Work out the finished part from the listing and answer in its coordinate system (mm). A direction names the side the tool comes from. Coordinates: 2 decimals unless noted, no trailing zeros. Order: outer loops, then holes, each group sorted by start corner. A loop starts at its lowest first (then second) coordinate and runs counter-clockwise, first axis right, second up.
1. The part is cut by section A-A, the plane y = -2.15. Give the vertices of the cut face in (x, z) (3 decimals).
2. The part is cut by section C-C, the plane y = -1.15. Give the vertices of the cut face in (x, z) (3 decimals).
3. Flat-ended cylindrical pins translate along their axes: pin 1 Ø2.5 at (x, z) = (-6, -1.5) entering from -Y; pin 2 Ø4 at (x, z) = (-3.5, 2) entering from +Y; pin 3 Ø1.6 at (x, y) = (-4.5, -1) entering from -Z. Find the tip coordinate at first contact, or state that the pin passes through.
4. The part is cut by section D-D, the plane x = -4.5. Give the vertices of the cut face in (y, z).
5. The part is cut by section B-B, the plane z = 1.25. Give the vertices of the cut face in (x, y).
6. A tool of negligible diameter and unlimited length cuts with its end or side. For faces 1 (the flat face through (-9, -1, -0.51)), 2 (the flat face through (-5.915, -1, -4)), 3 (the flat face through (-5.915, -1, 2)), from which of +Z, -Z, +X, -X, +Y, -Y can it reach the whole face along a straight path? Write none if from no direction.
7. Find the intervals of material crossed by probe 1 along Y at (x, z) = (-9.5, -2.25); probe 2 along X at (y, z) = (-1.45, -0.75); probe 3 along X at (y, z) = (-2.7, 0), in increasing order.
```python
from build123d import *

# Parameters (mm, degrees)
F1_DEPTH = 3
F0_W     = 0.8
F0_H     = 0.8
F2_DEPTH = 0.5
F3_DEPTH = 2


with BuildPart() as f1:
    # F0 (on Front) → F1 (new body)
    with BuildSketch(Plane.XZ):
        with BuildLine():
            Line((-6.7150478527, -4.8896004256), (-6.7150478527, -3.377443213))
            ThreePointArc((-6.7150478527, -3.377443213), (-8.0828148057, -2.6774176301), (-8.7828403885, -1.3096506771))
            Line((-8.7828403885, -1.3096506771), (-10.2949976011, -1.3096506771))
            ThreePointArc((-10.2949976011, -1.3096506771), (-9.1434749774, -3.7380778019), (-6.7150478527, -4.8896004256))
        make_face()
        with BuildLine():
            Line((-5.9150478527, -4.8896004256), (-5.9150478527, -3.377443213))
            ThreePointArc((-5.9150478527, -3.377443213), (-6.3150478527, -3.4096506771), (-6.7150478527, -3.377443213))
            Line((-6.7150478527, -3.377443213), (-6.7150478527, -4.8896004256))
            Line((-6.7150478527, -4.8896004256), (-5.9150478527, -4.8896004256))
        make_face()
        with BuildLine():
            Line((-2.3350981043, -1.3096506771), (-3.8472553168, -1.3096506771))
            ThreePointArc((-3.8472553168, -1.3096506771), (-4.5472808997, -2.6774176301), (-5.9150478527, -3.377443213))
            Line((-5.9150478527, -3.377443213), (-5.9150478527, -4.8896004256))
            ThreePointArc((-5.9150478527, -4.8896004256), (-3.4866207279, -3.7380778019), (-2.3350981043, -1.3096506771))
        make_face()
        with BuildLine():
            ThreePointArc((-3.8472553168, -0.5096506771), (-3.8231127272, -0.7090033991), (-3.8150478527, -0.9096506771))
            ThreePointArc((-3.8150478527, -0.9096506771), (-3.8231127272, -1.1102979552), (-3.8472553168, -1.3096506771))
            Line((-3.8472553168, -1.3096506771), (-2.3350981043, -1.3096506771))
            Line((-2.3350981043, -1.3096506771), (-2.3350981043, -0.5096506771))
            Line((-2.3350981043, -0.5096506771), (-3.8472553168, -0.5096506771))
        make_face()
        with BuildLine():
            ThreePointArc((-5.9150478527, 1.5581418587), (-4.5472808997, 0.8581162758), (-3.8472553168, -0.5096506771))
            Line((-3.8472553168, -0.5096506771), (-2.3350981043, -0.5096506771))
            ThreePointArc((-2.3350981043, -0.5096506771), (-3.4866207279, 1.9187764476), (-5.9150478527, 3.0702990713))
            Line((-5.9150478527, 3.0702990713), (-5.9150478527, 1.5581418587))
        make_face()
        with BuildLine():
            ThreePointArc((-6.7150478527, 1.5581418587), (-6.3150478527, 1.5903493229), (-5.9150478527, 1.5581418587))
            Line((-5.9150478527, 1.5581418587), (-5.9150478527, 3.0702990713))
            Line((-5.9150478527, 3.0702990713), (-6.7150478527, 3.0702990713))
            Line((-6.7150478527, 3.0702990713), (-6.7150478527, 1.5581418587))
        make_face()
        with BuildLine():
            ThreePointArc((-8.7828403885, -0.5096506771), (-8.0828148057, 0.8581162758), (-6.7150478527, 1.5581418587))
            Line((-6.7150478527, 1.5581418587), (-6.7150478527, 3.0702990713))
            ThreePointArc((-6.7150478527, 3.0702990713), (-9.1434749774, 1.9187764476), (-10.2949976011, -0.5096506771))
            Line((-10.2949976011, -0.5096506771), (-8.7828403885, -0.5096506771))
        make_face()
        with BuildLine():
            ThreePointArc((-8.7828403885, -1.3096506771), (-8.8150478527, -0.9096506771), (-8.7828403885, -0.5096506771))
            Line((-8.7828403885, -0.5096506771), (-10.2949976011, -0.5096506771))
            Line((-10.2949976011, -0.5096506771), (-10.2949976011, -1.3096506771))
            Line((-10.2949976011, -1.3096506771), (-8.7828403885, -1.3096506771))
        make_face()
        with BuildLine():
            Line((-6.7150478527, 3.0702990713), (-5.9150478527, 3.0702990713))
            ThreePointArc((-5.9150478527, 3.0702990713), (-6.3150478527, 3.0903493229), (-6.7150478527, 3.0702990713))
        make_face()
        with BuildLine():
            ThreePointArc((-2.3150478527, -0.9096506771), (-2.3200635603, -0.7093995769), (-2.3350981043, -0.5096506771))
            Line((-2.3350981043, -0.5096506771), (-2.3350981043, -1.3096506771))
            ThreePointArc((-2.3350981043, -1.3096506771), (-2.3200635603, -1.1099017774), (-2.3150478527, -0.9096506771))
        make_face()
        with BuildLine():
            Line((-10.2949976011, -1.3096506771), (-10.2949976011, -0.5096506771))
            ThreePointArc((-10.2949976011, -0.5096506771), (-10.3150478527, -0.9096506771), (-10.2949976011, -1.3096506771))
        make_face()
        with BuildLine():
            ThreePointArc((-6.7150478527, -4.8896004256), (-6.3150478527, -4.9096506771), (-5.9150478527, -4.8896004256))
            Line((-5.9150478527, -4.8896004256), (-6.7150478527, -4.8896004256))
        make_face()
    extrude(amount=F1_DEPTH)

    # F0 (on Front) → F2 (join)
    with BuildSketch(Plane.XZ):
        with BuildLine():
            ThreePointArc((-6.7150478527, -3.377443213), (-6.3150478527, -3.4096506771), (-5.9150478527, -3.377443213))
            Line((-5.9150478527, -3.377443213), (-5.9150478527, -1.3096506771))
            Line((-5.9150478527, -1.3096506771), (-6.7150478527, -1.3096506771))
            Line((-6.7150478527, -1.3096506771), (-6.7150478527, -3.377443213))
        make_face()
        with Locations((-6.3150478527, -0.9096506771)):
            Rectangle(F0_W, F0_H)
        with BuildLine():
            Line((-6.7150478527, -1.3096506771), (-6.7150478527, -0.5096506771))
            Line((-6.7150478527, -0.5096506771), (-8.7828403885, -0.5096506771))
            ThreePointArc((-8.7828403885, -0.5096506771), (-8.8150478527, -0.9096506771), (-8.7828403885, -1.3096506771))
            Line((-8.7828403885, -1.3096506771), (-6.7150478527, -1.3096506771))
        make_face()
        with BuildLine():
            Line((-5.9150478527, -0.5096506771), (-5.9150478527, 1.5581418587))
            ThreePointArc((-5.9150478527, 1.5581418587), (-6.3150478527, 1.5903493229), (-6.7150478527, 1.5581418587))
            Line((-6.7150478527, 1.5581418587), (-6.7150478527, -0.5096506771))
            Line((-6.7150478527, -0.5096506771), (-5.9150478527, -0.5096506771))
        make_face()
        with BuildLine():
            ThreePointArc((-3.8472553168, -1.3096506771), (-3.8231127272, -1.1102979552), (-3.8150478527, -0.9096506771))
            ThreePointArc((-3.8150478527, -0.9096506771), (-3.8231127272, -0.7090033991), (-3.8472553168, -0.5096506771))
            Line((-3.8472553168, -0.5096506771), (-5.9150478527, -0.5096506771))
            Line((-5.9150478527, -0.5096506771), (-5.9150478527, -1.3096506771))
            Line((-5.9150478527, -1.3096506771), (-3.8472553168, -1.3096506771))
        make_face()
    extrude(amount=F2_DEPTH)

    # F0 (on Front) → F3 (cut)
    with BuildSketch(Plane.XZ):
        with BuildLine():
            Line((-2.3350981043, -1.3096506771), (-3.8472553168, -1.3096506771))
            ThreePointArc((-3.8472553168, -1.3096506771), (-4.5472808997, -2.6774176301), (-5.9150478527, -3.377443213))
            Line((-5.9150478527, -3.377443213), (-5.9150478527, -4.8896004256))
            ThreePointArc((-5.9150478527, -4.8896004256), (-3.4866207279, -3.7380778019), (-2.3350981043, -1.3096506771))
        make_face()
        with BuildLine():
            Line((-6.7150478527, -4.8896004256), (-6.7150478527, -3.377443213))
            ThreePointArc((-6.7150478527, -3.377443213), (-8.0828148057, -2.6774176301), (-8.7828403885, -1.3096506771))
            Line((-8.7828403885, -1.3096506771), (-10.2949976011, -1.3096506771))
            ThreePointArc((-10.2949976011, -1.3096506771), (-9.1434749774, -3.7380778019), (-6.7150478527, -4.8896004256))
        make_face()
        with BuildLine():
            ThreePointArc((-8.7828403885, -0.5096506771), (-8.0828148057, 0.8581162758), (-6.7150478527, 1.5581418587))
            Line((-6.7150478527, 1.5581418587), (-6.7150478527, 3.0702990713))
            ThreePointArc((-6.7150478527, 3.0702990713), (-9.1434749774, 1.9187764476), (-10.2949976011, -0.5096506771))
            Line((-10.2949976011, -0.5096506771), (-8.7828403885, -0.5096506771))
        make_face()
        with BuildLine():
            ThreePointArc((-5.9150478527, 1.5581418587), (-4.5472808997, 0.8581162758), (-3.8472553168, -0.5096506771))
            Line((-3.8472553168, -0.5096506771), (-2.3350981043, -0.5096506771))
            ThreePointArc((-2.3350981043, -0.5096506771), (-3.4866207279, 1.9187764476), (-5.9150478527, 3.0702990713))
            Line((-5.9150478527, 3.0702990713), (-5.9150478527, 1.5581418587))
        make_face()
    extrude(amount=F3_DEPTH, mode=Mode.SUBTRACT)


solid = f1.part
```
Geometry says:
1. outline: circle Ø8 at (-6.315, -0.91); hole circle Ø5 at (-6.315, -0.91)
2. outline: (-10.295, -1.31) - (-8.783, -1.31) arc R2.5 cw to (-8.783, -0.51) - (-10.295, -0.51) arc R4 ccw to start; (-6.715, -4.89) arc R4 ccw to (-5.915, -4.89) - (-5.915, -3.377) arc R2.5 cw to (-6.715, -3.377) - close; (-6.715, 1.558) arc R2.5 cw to (-5.915, 1.558) - (-5.915, 3.07) arc R4 ccw to (-6.715, 3.07) - close; (-3.847, -1.31) - (-2.335, -1.31) arc R4 ccw to (-2.335, -0.51) - (-3.847, -0.51) arc R2.5 cw to start
3. pin 1: stops at y = -0.5
3. pin 2: stops at y = -2
3. pin 3: stops at z = -1.31
4. outline: (-3, -4.47) - (-2, -4.47) - (-2, -2.63) - (-3, -2.63) - close; (-3, 0.81) - (-2, 0.81) - (-2, 2.65) - (-3, 2.65) - close; (-0.5, -1.31) - (0, -1.31) - (0, -0.51) - (-0.5, -0.51) - close
5. outline: (-9.68, -3) - (-7.57, -3) - (-7.57, -2) - (-9.68, -2) - close; (-6.72, -0.5) - (-5.92, -0.5) - (-5.92, 0) - (-6.72, 0) - close; (-5.06, -3) - (-2.95, -3) - (-2.95, -2) - (-5.06, -2) - close
6. face 1: +Z, -X, +Y
6. face 2: -Z, +X, +Y
6. face 3: +Z, +X, +Y
7. probe 1: y = -3 to -2
7. probe 2: x = -10.31 to -8.81, -3.82 to -2.32
7. probe 3: x = -10.21 to -8.64, -3.99 to -2.42
